from build123d import *

# Parameters (mm, degrees)
SKETCH1_W         = 94
SKETCH1_H         = 190
PLATE_DEPTH       = 12
SKETCH2_R         = 17.5
BOSS_DEPTH        = 10
SKETCH3_R         = 11
CENTER_HOLE_DEPTH = 109.249711316
FILLET_R5_R       = 5
FILLET_R2_R       = 2


with BuildPart() as part:
    # Sketch1 → plate (new body)
    with BuildSketch(Plane(origin=(0, 0, 0), x_dir=(1, 0, 0), z_dir=(0, 1, 0))):
        Rectangle(SKETCH1_W, SKETCH1_H)
    extrude(amount=PLATE_DEPTH)

    # Sketch2 → boss (add)
    with BuildSketch(Plane(origin=(0, 12, 0), x_dir=(-1, 0, 0), z_dir=(0, 1, 0))):
        with Locations(Location((0, 0, 0), (0, 0, 270))):
            Circle(SKETCH2_R)
    extrude(amount=BOSS_DEPTH)

    # Sketch3 → center hole (cut, through all)
    with BuildSketch(Plane(origin=(0, 22, 0), x_dir=(-1, 0, 0), z_dir=(0, 1, 0))):
        with Locations(Location((0, 0, 0), (0, 0, 90))):
            Circle(SKETCH3_R)
    extrude(amount=-CENTER_HOLE_DEPTH, mode=Mode.SUBTRACT)

    # Sketch4 → pattern hole (revolve, cut)
    with BuildSketch(Plane(origin=(-35, 12, 80), x_dir=(0, 0, 1), z_dir=(1, 0, 0))):
        Polygon((0, 0), (0, 12), (4, 12), (4, 6.201721238), (6, 5), (6, 0), align=None)
    revolve(axis=Axis((-35, 18.130023899, 80), (0, -1, 0)), mode=Mode.SUBTRACT)

    # Fillet R5
    fillet_r5_edges = [part.edges().sort_by_distance(p)[0] for p in [
        (-47, 6, -95),
        (47, 6, -95),
        (47, 6, 95),
        (-47, 6, 95),
    ]]
    fillet(fillet_r5_edges, radius=FILLET_R5_R)

    # Fillet R2
    fillet_r2_edges = [part.edges().sort_by_distance(p)[0] for p in [
        (0, 12, 17.5),
        (0, 22, 17.5),
        (47, 12, 0),
        (0, 12, 95),
        (-47, 12, 0),
        (0, 12, -95),
        (45.535533906, 12, -93.535533906),
        (-45.535533906, 12, -93.535533906),
        (-45.535533906, 12, 93.535533906),
        (45.535533906, 12, 93.535533906),
    ]]
    fillet(fillet_r2_edges, radius=FILLET_R2_R)


solid = part.part
CAD build for the part. Positions are in the model's coordinates, mm. A direction names the side the tool comes from. Give positions to 0.01 mm unless a question says otherwise; leave off trailing zeros. Write each loop counter-clockwise with the first axis right and the second up, starting at its lowest first coordinate (ties: lowest second). Pieces come first, ordered by that corner, then holes. Notation, with made-up numbers: (-2, 82) -> (13, 82) arc R24 ccw to (13, 106) -> close; hole circle Ø6 at (42.5, 26.25). An arc over 180 degrees is marked (long way). Return JSON: item names as keys, results as strings.
Item 1: Drill centre lines: probe 1 along X at (y, z) = (1.95, 80); probe 2 along Z at (x, y) = (-35, 9.5); probe 3 along Y at (x, z) = (-18.5, -13). Where is each one in solid material? Low to high.
Answer below:
{"probe 1": "x = -47 to -39, -31 to 47", "probe 2": "z = -95 to 74, 86 to 95", "probe 3": "y = 0 to 12"}
Item 2: Band-saw the part on C-C (y = 18). List the corners of the cut face in (x, z), then the cut area to 3 significant figures.
Answer below:
{"outline": "circle Ø35 at (0, 0); hole circle Ø22 at (0, 0)", "area": "582 mm2"}
Item 3: Drop flat-ended pins along their axis: pin 1 (10 mm diameter, centred on x = 31, z = -43.5, fed in from +Y); pin 2 (5 mm diameter, centred on x = -12, y = 15.5, fed in from +Z); pin 3 (9.5 mm diameter, centred on x = -35, z = 80, fed in from +Y); pin 4 (13 mm diameter, centred on x = 0, z = 0, fed in from +Y). Give the stop position or say it passes through.
Answer below:
{"pin 1": "stops at y = 12", "pin 2": "stops at z = 14.7", "pin 3": "stops at y = 6.25", "pin 4": "passes through"}
Item 4: Band-saw the part on B-B (x = -35). List the corners of the cut face in (y, z), then the cut area to 3 significant figures.
Answer below:
{"outline": "(0, -95) -> (10, -95) arc R2 ccw to (12, -93) -> (12, 74) -> (7, 74) -> (5.8, 76) -> (0, 76) -> close; (0, 84) -> (5.8, 84) -> (7, 86) -> (12, 86) -> (12, 93) arc R2 ccw to (10, 95) -> (0, 95) -> close", "area": "2,160 mm2"}
Item 5: Two-plate mould, pull along X, no slides. Class faces 3 (the cylindrical face through (-35, 10, 74)), 4 (the flat face through (-1, 12, -22)), 5 (the cylindrical face through (-38.966, 2.94, 79.479)), 6 (the cylindrical face through (-46, 5, -93)): +X half, -X half, draft (parallel to the pull), parting line (faces both ways), or undercut.
Answer below:
{"face 3": "undercut", "face 4": "draft", "face 5": "undercut", "face 6": "-X half"}
Item 6: Band-saw the part on D-D (z = -42). List the corners of the cut face in (x, y), then the cut area to 3 significant figures.
Answer below:
{"outline": "(-47, 0) -> (47, 0) -> (47, 10) arc R2 ccw to (45, 12) -> (-45, 12) arc R2 ccw to (-47, 10) -> close", "area": "1,130 mm2"}
Item 7: Band-saw the part on A-A (z = 0). List the corners of the cut face in (x, y), then the cut area to 3 significant figures.
Answer below:
{"outline": "(-47, 0) -> (-11, 0) -> (-11, 22) -> (-15.5, 22) arc R2 ccw to (-17.5, 20) -> (-17.5, 14) arc R2 cw to (-19.5, 12) -> (-45, 12) arc R2 ccw to (-47, 10) -> close; (11, 0) -> (47, 0) -> (47, 10) arc R2 ccw to (45, 12) -> (19.5, 12) arc R2 cw to (17.5, 14) -> (17.5, 20) arc R2 ccw to (15.5, 22) -> (11, 22) -> close", "area": "992 mm2"}
Item 8: Tool access for faces 1 (the flat face through (-1, 5, -95)), 2 (the cylindrical face through (10.648, 16.958, 13.887)): list every direction of +Z, -Z, +X, -X, +Y, -Y with a clear straight run to the whole face (end or side of a thin tool).
Answer below:
{"face 1": "-Z, +X, -X, +Y, -Y", "face 2": "+Y"}
